CAD build for the part. Positions are in the model's coordinates, mm. A direction names the side the tool comes from. Round coordinates to 2 decimals unless told otherwise and drop trailing zeros. Loops run counter-clockwise (first coordinate to the right, second up) from the corner with the lowest first, then second, coordinate; pieces in that order, holes last. Notation, with made-up numbers: M 18,24 L 72,24 A20 ccw 72,41 Z; hole C -7.5,-14.75 d9. An arc over 180 degrees is marked long. One line per item, written item: value. Start each with the question number.
from build123d import *

# Parameters (mm, degrees)
F0_R     = 38.1
F1_DEPTH = 31.75
F2_R     = 5.08
F3_R     = 19.05
F4_DEPTH = 101.6
F5_R     = 38.1
F6_DEPTH = 31.75
F7_R     = 5.08


with BuildPart() as f1:
    # F0 (on Right) → F1 (new body)
    with BuildSketch(Plane.YZ):
        Circle(F0_R)
    extrude(amount=F1_DEPTH)

    # F2
    f2_edges = [f1.edges().sort_by_distance(p)[0] for p in [
        (0, -38.1, 0),
        (31.75, -38.1, 0),
    ]]
    fillet(f2_edges, radius=F2_R)

    # F3 (on face) → F4 (join)
    with BuildSketch(Plane(origin=(0, 0, 0), x_dir=(0, -1, 0), z_dir=(-1, 0, 0))):
        Circle(F3_R)
    extrude(amount=F4_DEPTH)

    # F5 (on face) → F6 (join)
    with BuildSketch(Plane(origin=(-101.6, 0, 0), x_dir=(0, -1, 0), z_dir=(-1, 0, 0))):
        Circle(F5_R)
    extrude(amount=F6_DEPTH)

    # F7
    f7_edges = [f1.edges().sort_by_distance(p)[0] for p in [
        (-101.6, 38.1, 0),
        (-133.35, 38.1, 0),
    ]]
    fillet(f7_edges, radius=F7_R)


solid = f1.part
(1) Mould opens along X. For faces 3 (the flat face through (-133.35, 0, 0)), 4 (the flat face through (0, 14, -14)), 5 (the cylindrical face through (15.724, -30.235, -23.183)) say: pulls with the +X half, pulls with the -X half, needs draft (parallel to the pull), parting line crosses it, or undercut.
(2) Which spindle directions (+Z, -Z, +X, -X, +Y, -Y) get a long thin tool onto all of the face, cutting with end or side? Do faces 1 (the flat face through (31.75, 0, 0)), 2 (the flat face through (-101.6, -14, -14)). Say none if no direction does.
(3) Slice it at A-A, the plane z = 0. List the corners of the cut face in (x, y), and give its area (3 significant figures).
(4) Flat gauge pins, fed straight in: P1, Ø6, axis at x = -71.5, y = -2, coming from the -Z side; P2, Ø12, axis at x = -45, z = 7.5, coming from the -Y side; P3, Ø10, axis at x = -48, y = -11.5, coming from the -Z side. Where does each tip first touch, or does it go through?
(5) Slice it at C-C, the plane x = -16. List the corners of the cut face in (y, z).
(6) Slice it at D-D, the plane x = 22. List the corners of the cut face in (y, z), and give its area (3 significant figures).
(7) Probe L1, parallel to X at y = -14.5, z = -15; L2, parallel to X at y = 8.5, z = 33; L3, parallel to Z at x = 5, y = -11.5. List the from-to ranges inside material, lowest first.
Check result:
1. face 3: pulls with the -X half
1. face 4: undercut
1. face 5: needs draft
2. face 1: +Z, -Z, +X, +Y, -Y
2. face 2: none
3. outline: M -133.35,-33.02 A5.08 ccw -128.27,-38.1 L -106.68,-38.1 A5.08 ccw -101.6,-33.02 L -101.6,-19.05 L 0,-19.05 L 0,-33.02 A5.08 ccw 5.08,-38.1 L 26.67,-38.1 A5.08 ccw 31.75,-33.02 L 31.75,33.02 A5.08 ccw 26.67,38.1 L 5.08,38.1 A5.08 ccw 0,33.02 L 0,19.05 L -101.6,19.05 L -101.6,33.02 A5.08 ccw -106.68,38.1 L -128.27,38.1 A5.08 ccw -133.35,33.02 Z
3. area: 8,670 mm^2
4. P1: stops at z = -19.05
4. P2: stops at y = -18.99
4. P3: stops at z = -17.91
5. outline: C 0,0 d38.1
6. outline: C 0,0 d76.2
6. area: 4,560 mm^2
7. L1: x = -133.35 to -101.6, 0 to 31.75
7. L2: x = -133.24 to -101.71, 0.11 to 31.64
7. L3: z = -36.32 to 36.32
